```python
from build123d import *

# Parameters (mm, degrees)
SKETCH011_W           = 23.1
SKETCH011_H           = 23.1
PAD007_DEPTH          = 5
PAD008_DEPTH          = 2.8
POLARPATTERN001_COUNT = 4
SKETCH013_R           = 10.5
PAD009_DEPTH          = 9
PAD009_TAPER          = 2
SKETCH014_R           = 4
POCKET003_DEPTH       = 10
CHAMFER003_SIZE       = 1
CHAMFER_SIZE          = 2


with BuildPart() as part:
    # Sketch011 → Pad007 (new body)
    with BuildSketch(Plane.XY):
        Rectangle(SKETCH011_W, SKETCH011_H)
    extrude(amount=PAD007_DEPTH)

    # Sketch012 → Pad008 (join)
    with BuildSketch(Plane.XY):
        Polygon((0, 11.55), (1.8, 11.55), (1.8, 1.8), (11.55, 1.8), (11.55, 0), (0, 0), align=None)
    pad008 = extrude(amount=-PAD008_DEPTH)

    # PolarPattern001: Pad008 ×4 about axis
    polarpattern001_axis = Axis((0, 0, 0), (0, 0, 1))
    for i in range(1, POLARPATTERN001_COUNT):
        add(pad008.rotate(polarpattern001_axis, i * 360 / POLARPATTERN001_COUNT))

    # Sketch013 → Pad009 (join)
    with BuildSketch(Plane.XY):
        Circle(SKETCH013_R)
    extrude(amount=-PAD009_DEPTH, taper=PAD009_TAPER)

    # Sketch014 → Pocket003 (cut)
    with BuildSketch(Plane.XY.offset(-5)):
        Circle(SKETCH014_R)
    extrude(amount=POCKET003_DEPTH, mode=Mode.SUBTRACT)

    # Chamfer003
    chamfer003_edges = [part.edges().sort_by_distance(p)[0] for p in [
        (-11.55, -11.55, 2.5),
        (11.55, -11.55, 2.5),
        (-11.55, 11.55, 2.5),
        (11.55, 11.55, 2.5),
    ]]
    chamfer(chamfer003_edges, length=CHAMFER003_SIZE)

    # Chamfer
    chamfer_edges = [part.edges().sort_by_distance(p)[0] for p in [
        (-4, 0, 5),
    ]]
    chamfer(chamfer_edges, length=CHAMFER_SIZE)


solid = part.part
```
Could you check a few things on this model? Use its own coordinates, in mm. A direction names the side the tool comes from. Coordinates: 2 decimals unless noted, no trailing zeros. Order: outer loops, then holes, each group sorted by start corner. A loop starts at its lowest first (then second) coordinate and runs counter-clockwise, first axis right, second up. Notation, with made-up numbers: M -0.75,71 L 42.25,71 A12 ccw 42.25,88 Z; hole C -23.5,44 d6. An arc over 180 degrees is marked long. Use a Markdown table: item, result. Add a question column.
Q1. I'm going to push flat-ended pins straight in: pin 1 (1 mm diameter, centred on x = 0, y = 11, fed in from -Z); pin 2 (8 mm diameter, centred on y = -3.5, z = -7, fed in from +X); pin 3 (1 mm diameter, centred on x = 11, z = -1.5, fed in from +Y); pin 4 (6 mm diameter, centred on x = 9, y = 8.5, fed in from -Z). Where does each tip first touch, or does it pass through?
Q2. I want a section at A-A on x = 0. List the corners of the cut face in (y, z) for me.
Q3. We'd pull the mould along Y, two halves only. Please class faces 6 (the flat face through (-11, 0, -2.8)), 7 (the cylindrical face through (-0.867, -3.905, -1.056)), 8 (the flat face through (-11.1, -11, 2.5)): pulls with the +Y half, pulls with the -Y half, needs draft (parallel to the pull), parting line crosses it, or undercut.
Q4. I want a section at B-B on z = -1. List the corners of the cut face in (x, y) for me.
Q5. Which directions (+Z, -Z, +X, -X, +Y, -Y) give clear straight access to the entire face, cutting with the end or side of a thin tool? Please do faces 1 (the flat face through (11, 1.8, -1)), 2 (the flat face through (-1.8, -11, -1)), 3 (the flat face through (-11, 1.8, -1)), 4 (the flat face through (9, -9, 0)), 5 (the flat face through (0, 0, -9)).
Q6. I want a section at D-D on z = -7.25. List the corners of the cut face in (x, y) for me, then the cut area to 3 significant figures.
Q7. If I drill on L1, parallel to Y at x = 0, z = 1; L2, parallel to Z at x = -1.25, y = -1; L3, parallel to Z at x = -5.25, y = 10.25, over which ranges is the centre line in solid material (lowest first)?
Q8. I want a section at C-C on z = -2.5. List the corners of the cut face in (x, y) for me.
Checked values:
| question | item | result |
|---|---|---|
| 1 | pin 1 | z = -2.8 |
| 1 | pin 2 | x = 10.34 |
| 1 | pin 3 | y = 1.8 |
| 1 | pin 4 | z = -9 |
| 2 | outline | M -11.55,-2.8 L -10.4,-2.8 L -10.19,-9 L 10.19,-9 L 10.4,-2.8 L 11.55,-2.8 L 11.55,5 L 6,5 L 4,3 L 4,-5 L -4,-5 L -4,3 L -6,5 L -11.55,5 Z |
| 3 | face 6 | needs draft |
| 3 | face 7 | undercut |
| 3 | face 8 | pulls with the -Y half |
| 4 | outline | M -11.55,-1.8 L -10.31,-1.8 A10.47 ccw -1.8,-10.31 L -1.8,-11.55 L 1.8,-11.55 L 1.8,-10.31 A10.47 ccw 10.31,-1.8 L 11.55,-1.8 L 11.55,1.8 L 10.31,1.8 A10.47 ccw 1.8,10.31 L 1.8,11.55 L -1.8,11.55 L -1.8,10.31 A10.47 ccw -10.31,1.8 L -11.55,1.8 Z; hole C 0,0 d8 |
| 5 | face 1 | -Z, +X, +Y |
| 5 | face 2 | -Z, -X, -Y |
| 5 | face 3 | -Z, -X, +Y |
| 5 | face 4 | -Z, +X, -Y |
| 5 | face 5 | -Z, +X, -X, +Y, -Y |
| 6 | outline | C 0,0 d20.49 |
| 6 | area | 330 mm² |
| 7 | L1 | -11.55 to -4, 4 to 11.55 |
| 7 | L2 | -9 to -5 |
| 7 | L3 | 0 to 5 |
| 8 | outline | M -11.55,-1.8 L -10.26,-1.8 A10.41 ccw -1.8,-10.26 L -1.8,-11.55 L 1.8,-11.55 L 1.8,-10.26 A10.41 ccw 10.26,-1.8 L 11.55,-1.8 L 11.55,1.8 L 10.26,1.8 A10.41 ccw 1.8,10.26 L 1.8,11.55 L -1.8,11.55 L -1.8,10.26 A10.41 ccw -10.26,1.8 L -11.55,1.8 Z; hole C 0,0 d8 |
